Design review of the part built by this model. Coordinates are the model's own, in mm. Face numbers are marked on the shaded views. A direction names the side the tool comes from. Give positions to 0.01 mm unless a question says otherwise; leave off trailing zeros. Order: outer loops, then holes, each group sorted by start corner. A loop starts at its lowest first (then second) coordinate and runs counter-clockwise, first axis right, second up. Notation, with made-up numbers: M 64.25,49.5 L 92.25,49.5 A34 ccw 92.25,82.5 Z; hole C 33.25,7.5 d8. An arc over 180 degrees is marked long. Answer as a JSON object with one key per item and string values.
from build123d import *

# Parameters (mm, degrees)
SKETCH1_W            = 26.1
SKETCH1_H            = 27.1
SKETCH1_W_2          = 13
SKETCH1_H_2          = 12.5
BOSS_EXTRUDE1_DEPTH  = 1
BOSS_EXTRUDE2_DEPTH  = 4
SKETCH3_W            = 1
SKETCH3_H            = 24.1
BOSS_EXTRUDE3_DEPTH  = 3
BOSS_EXTRUDE4_DEPTH  = 3
FILLET1_R            = 0.3
BOSS_EXTRUDE5_DEPTH  = 6
FILLET2_R            = 0.3
FILLET2_OF_MIRROR2_R = 0.3
SKETCH8_W            = 13
SKETCH8_H            = 12.5
SKETCH8_W_2          = 12.7
SKETCH8_H_2          = 12.2
BOSS_EXTRUDE6_DEPTH  = 1
SKETCH14_W           = 6
SKETCH14_H           = 3.7
BOSS_EXTRUDE8_DEPTH  = 3.45
SKETCH15_R           = 1.35
CUT_EXTRUDE4_DEPTH   = 0.7
FILLET6_R            = 0.3
CUT_EXTRUDE5_DEPTH   = 0.4
FILLET7_R            = 3
MIRROR4_START        = -2.2
MIRROR4_2_OUTLINE_W  = 2.3
MIRROR4_2_OUTLINE_H  = 0.4
MIRROR4_2_DEPTH      = 2.7
FILLET8_R            = 1
CHAMFER1_SIZE        = 0.5
CHAMFER2_SIZE        = 0.5


with BuildPart() as part:
    # Sketch1 → Boss-Extrude1 (new body)
    with BuildSketch(Plane(origin=(0, 0, 0), x_dir=(1, 0, 0), z_dir=(0, 1, 0))):
        with Locations((5.25, 6.25)):
            Rectangle(SKETCH1_W, SKETCH1_H)
        with Locations((6.5, 6.25)):
            Rectangle(SKETCH1_W_2, SKETCH1_H_2, mode=Mode.SUBTRACT)
    extrude(amount=BOSS_EXTRUDE1_DEPTH)

    # Sketch2 → Boss-Extrude2 (add)
    with BuildSketch(Plane.XZ):
        Polygon((-7.8, 7.3), (-7.8, -19.8), (18.3, -19.8), (18.3, -18.3), (17.3, -18.3), (17.3, -18.8), (-6.8, -18.8), (-6.8, 6.3), (17.3, 6.3), (17.3, 5.8), (18.3, 5.8), (18.3, 7.3), align=None)
    extrude(amount=BOSS_EXTRUDE2_DEPTH)

    # Sketch3 → Boss-Extrude3 (add)
    with BuildSketch(Plane.XZ):
        with Locations((17.8, -6.25)):
            Rectangle(SKETCH3_W, SKETCH3_H)
    extrude(amount=BOSS_EXTRUDE3_DEPTH)

    # Sketch4 → Boss-Extrude4 (add, symmetric)
    with BuildSketch(Plane.XY.offset(-12.5)):
        Polygon((-6.8, -4), (-6.25, -3.570292905), (-6.8, -3.4), align=None)
    extrude(amount=BOSS_EXTRUDE4_DEPTH, both=True)

    # Fillet1
    # the kernel refuses this fillet: 0.3 mm, written as the material it adds along each edge
    with BuildSketch(Plane(origin=(-6.8, -2.65, -15.5), x_dir=(0, 0, -1), z_dir=(0, -1, 0))) as fillet1_piece_1_section:
        with BuildLine():
            CenterArc((FILLET1_R, FILLET1_R), FILLET1_R, 180, 90)
            Line((0, FILLET1_R), (0, 0))
            Line((0, 0), (FILLET1_R, 0))
        make_face()
    fillet1_piece_1 = extrude(amount=1.35, mode=Mode.PRIVATE)
    fillet1_piece_1 = split(fillet1_piece_1, bisect_by=Plane(origin=(-7.011903145, -3.334389814, -15.5), z_dir=(-0.2957706001702403, -0.9552589973797346, 0)), keep=Keep.TOP, mode=Mode.PRIVATE)
    fillet1_piece_1 = split(fillet1_piece_1, bisect_by=Plane(origin=(-6.145050385, -3.48829728, -15.5), z_dir=(-0.6156614753256621, 0.7880107536067191, 0)), keep=Keep.TOP, mode=Mode.PRIVATE)
    add(fillet1_piece_1)
    with BuildSketch(Plane(origin=(-6.8, -2.65, -9.5), x_dir=(0, 0, 1), z_dir=(0, -1, 0))) as fillet1_piece_2_section:
        with BuildLine():
            CenterArc((FILLET1_R, -FILLET1_R), FILLET1_R, 90, 90)
            Line((0, -FILLET1_R), (0, 0))
            Line((0, 0), (FILLET1_R, 0))
        make_face()
    fillet1_piece_2 = extrude(amount=1.35, mode=Mode.PRIVATE)
    fillet1_piece_2 = split(fillet1_piece_2, bisect_by=Plane(origin=(-7.011903145, -3.334389814, -9.5), z_dir=(-0.2957706001702403, -0.9552589973797346, 0)), keep=Keep.TOP, mode=Mode.PRIVATE)
    fillet1_piece_2 = split(fillet1_piece_2, bisect_by=Plane(origin=(-6.145050385, -3.48829728, -9.5), z_dir=(-0.6156614753256621, 0.7880107536067191, 0)), keep=Keep.TOP, mode=Mode.PRIVATE)
    add(fillet1_piece_2)

    # Sketch6 → Boss-Extrude5 (add)
    with BuildSketch(Plane.ZY.offset(-13)):
        Polygon((-18.8, -4), (-18.25, -3.570292905), (-18.8, -3.4), align=None)
    boss_extrude5 = extrude(amount=BOSS_EXTRUDE5_DEPTH)

    # Fillet2
    fillet2_edges = [part.edges().sort_by_distance(p)[0] for p in [
        (13, -3.7, -18.8),
        (7, -3.7, -18.8),
    ]]
    fillet(fillet2_edges, radius=FILLET2_R)

    # Mirror2: Boss-Extrude5 across plane
    add(boss_extrude5.mirror(Plane(origin=(0, 0, -6.25), x_dir=(1, 0, 0), z_dir=(0, 0, -1))))

    # Fillet2 of Mirror2
    fillet2_of_mirror2_edges = [part.edges().sort_by_distance(p)[0] for p in [
        (13, -3.7, 6.3),
        (7, -3.7, 6.3),
    ]]
    fillet(fillet2_of_mirror2_edges, radius=FILLET2_OF_MIRROR2_R)

    # Sketch8 → Boss-Extrude6 (add)
    with BuildSketch(Plane(origin=(0, 1, 0), x_dir=(1, 0, 0), z_dir=(0, 1, 0))):
        with Locations((6.5, 6.25)):
            Rectangle(SKETCH8_W, SKETCH8_H)
        with Locations((6.5, 6.25)):
            Rectangle(SKETCH8_W_2, SKETCH8_H_2, mode=Mode.SUBTRACT)
    extrude(amount=-BOSS_EXTRUDE6_DEPTH)

    # Sketch14 → Boss-Extrude8 (add, symmetric)
    with BuildSketch(Plane(origin=(0, 0, -6.25), x_dir=(-1, 0, 0), z_dir=(0, 0, -1))):
        with Locations((10.8, -0.85)):
            Rectangle(SKETCH14_W, SKETCH14_H)
    extrude(amount=BOSS_EXTRUDE8_DEPTH, both=True)

    # Sketch15 → Cut-Extrude4 (cut)
    with BuildSketch(Plane(origin=(0, 0, -9.7), x_dir=(-1, 0, 0), z_dir=(0, 0, -1))):
        with Locations((11.5, -0.85)):
            Circle(SKETCH15_R)
    extrude(amount=-CUT_EXTRUDE4_DEPTH, mode=Mode.SUBTRACT)

    # Fillet6
    fillet6_edges = [part.edges().sort_by_distance(p)[0] for p in [
        (-10.15, -0.85, -9),
    ]]
    fillet(fillet6_edges, radius=FILLET6_R)

    # Sketch16 → Cut-Extrude5 (cut)
    with BuildSketch(Plane(origin=(0, 0, -9.7), x_dir=(-1, 0, 0), z_dir=(0, 0, -1))):
        with BuildLine():
            Line((13.8, 0.5), (11.5, 0.5))
            ThreePointArc((11.5, 0.5), (12.454594155, 0.104594155), (12.85, -0.85))
            ThreePointArc((12.85, -0.85), (12.454594155, -1.804594155), (11.5, -2.2))
            Line((11.5, -2.2), (13.8, -2.2))
            Line((13.8, -2.2), (13.8, 0.5))
        make_face()
    extrude(amount=-CUT_EXTRUDE5_DEPTH, mode=Mode.SUBTRACT)

    # Fillet7
    # the kernel refuses this fillet: 3 mm, written as the material it adds along each edge
    with BuildSketch(Plane(origin=(-7.8, -2.7, -2.8), x_dir=(-1, 0, 0), z_dir=(0, 0, -1))) as fillet7_piece_1:
        with BuildLine():
            CenterArc((2.471841419, -3), FILLET7_R, 90, 55.481892159)
            Line((0, -1.3), (-0.049436828, -1.266))
            ThreePointArc((-0.049436828, -1.266), (-0.06, -0.65), (-0.06, 0))
            Line((-0.06, 0), (0, 0.06))
            Line((0, 0.06), (2.471841419, 0.06))
            Line((2.471841419, 0.06), (2.471841419, 0))
        make_face()
    extrude(amount=6.9)

    # Mirror4: read off the stored shape, not the designer's step
    # Mirror4 outline → Mirror4 (revolve, cut)
    with BuildSketch(Plane(origin=(-11.5, -0.85, 0), x_dir=(1, 0, 0), z_dir=(0, -1, 0))):
        with BuildLine():
            Line((0, -2.8), (0, -3.5))
            Line((0, -3.5), (1.05, -3.5))
            ThreePointArc((1.05, -3.5), (1.262132034, -3.412132034), (1.35, -3.2))
            Line((1.35, -3.2), (1.35, -2.8))
            Line((1.35, -2.8), (0, -2.8))
        make_face()
    revolve(axis=Axis((-11.5, -0.85, 0), (0, 0, 1)), mode=Mode.SUBTRACT)

    # Mirror4 2 outline → Mirror4 2 (cut)
    with BuildSketch(Plane(origin=(0, 0, 0), x_dir=(1, 0, 0), z_dir=(0, 1, 0)).offset(MIRROR4_START)):
        with Locations((-12.65, 3)):
            Rectangle(MIRROR4_2_OUTLINE_W, MIRROR4_2_OUTLINE_H)
    extrude(amount=MIRROR4_2_DEPTH, mode=Mode.SUBTRACT)

    # Fillet8
    fillet8_edges = [part.edges().sort_by_distance(p)[0] for p in [
        (-13.8, 1, -6.25),
        (-13.8, -2.7, -6.25),
    ]]
    fillet(fillet8_edges, radius=FILLET8_R)

    # Chamfer1
    chamfer1_edges = [part.edges().sort_by_distance(p)[0] for p in [
        (-7.8, 1, -14.75),
        (5.25, 1, 7.3),
        (18.3, -1.5, -19.8),
        (18.3, -1.5, 7.3),
        (-7.8, -1.5, 7.3),
        (-7.8, -1.5, -19.8),
        (6.5, 1, -0.15),
        (12.85, 1, -6.25),
        (6.5, 1, -12.35),
        (0.15, 1, -6.25),
        (18.3, 1, -6.25),
        (-7.8, 1, 2.25),
        (-7.8, -4, -14.75),
        (-7.8, -4, 2.25),
        (5.25, 1, -19.8),
    ]]
    chamfer(chamfer1_edges, length=CHAMFER1_SIZE)

    # Chamfer2
    chamfer2_edges = [part.edges().sort_by_distance(p)[0] for p in [
        (-7.8, -1.5, -2.8),
        (-7.8, -1.5, -9.7),
    ]]
    chamfer(chamfer2_edges, length=CHAMFER2_SIZE)


solid = part.part
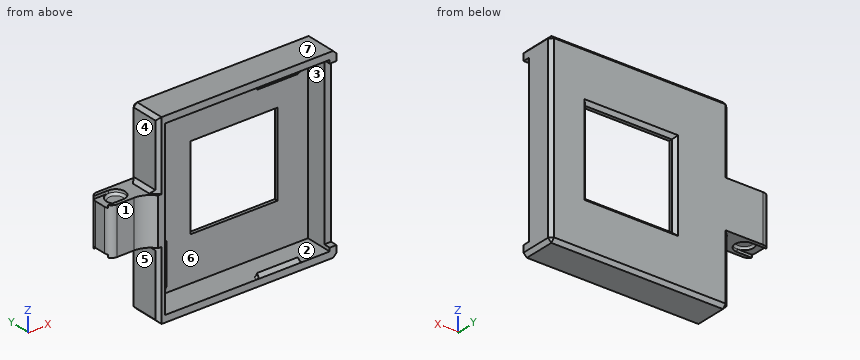
(1) We need section C-C (z = -1.5). Write out the cut boundary in (x, y), plus the area to 3 significant figures.
Checked values:
{"outline": "M -7.8,-3.5 L -7.3,-4 L -6.8,-4 L -6.8,0 L 0.15,0 L 0.15,0.5 L -0.35,1 L -7.3,1 L -7.8,0.5 Z; M 12.85,0 L 17.3,0 L 17.3,-3 L 18.3,-3 L 18.3,0.5 L 17.8,1 L 13.35,1 L 12.85,0.5 Z", "area": "19.8 mm^2"}
(2) Draft analysis for pull direction X (two halves, no side actions). For the marked faces 5, 6 and 7, state which applies: +X half, -X half, draft (parallel to the pull), parting line (faces both ways), or undercut.
Checked values:
{"face 5": "-X half", "face 6": "undercut", "face 7": "draft"}
(3) Tool access review of the marked faces 1, 2, 3 and 4: name each direction out of +Z, -Z, +X, -X, +Y, -Y from which nothing blocks a thin tool from reaching the whole face with its end or side.
Checked values:
{"face 1": "+Z, -Z, -X, -Y", "face 2": "none", "face 3": "-Y", "face 4": "+Z, -X, +Y, -Y"}
(4) To check wall thickness, follow L1, parallel to X at y = -0.85, z = -16.5; L2, parallel to Z at x = 4, y = -2.7; L3, parallel to Z at x = 8, y = 0.4. State the ranges of each line that lie inside material, in increasing order. Write a range as from..to.
Checked values:
{"L1": "x = -7.8..-6.8, 17.3..18.3", "L2": "z = -19.8..-18.8, 6.3..7.3", "L3": "z = -19.8..-12.35, -0.15..7.3"}
(5) We need section B-B (x = 12.5). Write out the cut boundary in (y, z), plus the area to 3 significant figures.
Checked values:
{"outline": "M -4,-19.8 L 0.5,-19.8 L 1,-19.3 L 1,-12.85 L 0.5,-12.35 L 0,-12.35 L 0,-18.8 L -3.4,-18.8 L -3.57,-18.25 L -4,-18.8 Z; M -4,6.3 L -3.57,5.75 L -3.4,6.3 L 0,6.3 L 0,-0.15 L 0.5,-0.15 L 1,0.35 L 1,6.8 L 0.5,7.3 L -4,7.3 Z", "area": "22.7 mm^2"}
(6) Insertion check: pin 1 (3 mm diameter, centred on y = -2, z = -6, fed in from -X); pin 2 (5 mm diameter, centred on x = 2, z = -5, fed in from -Y); pin 3 (1 mm diameter, centred on x = -11, y = -0.5, fed in from -Z); pin 4 (1.3 mm diameter, centred on x = -11, z = -8, fed in from -Y). Each pin has a flat end and moves straight along its axis. Give the tip position at first contact, or say it passes through.
Checked values:
{"pin 1": "stops at x = -13.8", "pin 2": "stops at y = 0", "pin 3": "stops at z = -9.01", "pin 4": "stops at y = -2.7"}
(7) We need section A-A (y = -0.85). Write out the cut boundary in (x, z).
Checked values:
{"outline": "M -13.8,-9.3 L -12.85,-9.3 A0.3 cw -12.55,-9 L -10.45,-9 A0.3 cw -10.15,-9.3 L -10.15,-9.7 L -8.3,-9.7 L -7.8,-10.2 L -7.8,-19.3 L -7.3,-19.8 L 17.8,-19.8 L 18.3,-19.3 L 18.3,6.8 L 17.8,7.3 L -7.3,7.3 L -7.8,6.8 L -7.8,-2.3 L -8.3,-2.8 L -10.15,-2.8 L -10.15,-3.2 A0.3 cw -10.45,-3.5 L -12.55,-3.5 A0.3 cw -12.85,-3.2 L -13.8,-3.2 Z; hole M -6.8,-18.8 L 17.3,-18.8 L 17.3,6.3 L -6.8,6.3 Z"}
(8) We need section D-D (z = 3.5). Write out the cut boundary in (x, y), plus the area to 3 significant figures.
Checked values:
{"outline": "M -7.8,-3.5 L -7.3,-4 L -6.8,-4 L -6.8,0 L 17.3,0 L 17.3,-3 L 18.3,-3 L 18.3,0.5 L 17.8,1 L -7.3,1 L -7.8,0.5 Z", "area": "32.7 mm^2"}
